```python
from build123d import *

# Parameters (mm, degrees)
BOSS_EXTRU_1_DEPTH   = 635
ESQUISSE2_R          = 486.41
BOSS_EXTRU_2_DEPTH   = 203.2
PER_AGE1_D           = 139.7
PER_AGE1_DEPTH       = 838.2
PER_AGE1_CBORE_D     = 266.7
PER_AGE1_CBORE_DEPTH = 165.1
PER_AGE2_D           = 139.7
PER_AGE2_DEPTH       = 838.2
PER_AGE2_CBORE_D     = 292.1
PER_AGE2_CBORE_DEPTH = 165.1


with BuildPart() as part:
    # Esquisse1 → Boss.-Extru.1 (new body)
    with BuildSketch(Plane.XY.offset(838.2)):
        with BuildLine():
            ThreePointArc((-720.101782381, 451.601786597), (-655.471932336, 350.063866609), (-659.625858178, 229.773752251))
            ThreePointArc((-659.625858178, 229.773752251), (-493.914086659, -493.914086659), (229.773752251, -659.625858178))
            ThreePointArc((229.773752251, -659.625858178), (350.063866609, -655.471932336), (451.601786597, -720.101782381))
            ThreePointArc((451.601786597, -720.101782381), (731.603841816, -731.603841816), (720.101782381, -451.601786597))
            ThreePointArc((720.101782381, -451.601786597), (655.471932336, -350.063866609), (659.625858178, -229.773752251))
            ThreePointArc((659.625858178, -229.773752251), (493.914086659, 493.914086659), (-229.773752251, 659.625858178))
            ThreePointArc((-229.773752251, 659.625858178), (-350.063866609, 655.471932336), (-451.601786597, 720.101782381))
            ThreePointArc((-451.601786597, 720.101782381), (-731.603841816, 731.603841816), (-720.101782381, 451.601786597))
        make_face()
    extrude(amount=-BOSS_EXTRU_1_DEPTH)

    # Esquisse2 → Boss.-Extru.2 (add)
    with BuildSketch(Plane(origin=(0, 0, 203.2), x_dir=(-1, 0, 0), z_dir=(0, 0, -1))):
        Circle(ESQUISSE2_R)
    extrude(amount=BOSS_EXTRU_2_DEPTH)

    # Perçage1
    with Locations(Plane.XY.offset(838.2)):
        with Locations((-596.9, 596.9)):
            CounterBoreHole(PER_AGE1_D / 2, PER_AGE1_CBORE_D / 2, PER_AGE1_CBORE_DEPTH, depth=PER_AGE1_DEPTH)

    # Perçage2
    with Locations(Plane.XY.offset(838.2)):
        with Locations((596.9, -596.9)):
            CounterBoreHole(PER_AGE2_D / 2, PER_AGE2_CBORE_D / 2, PER_AGE2_CBORE_DEPTH, depth=PER_AGE2_DEPTH)


solid = part.part
```
Input: part model. Units: mm. Frame: model coordinates. A direction names the side the tool comes from. Coordinates: 2 decimals unless noted, no trailing zeros. Write each loop counter-clockwise with the first axis right and the second up, starting at its lowest first coordinate (ties: lowest second). Pieces come first, ordered by that corner, then holes.
1) Section A-A on x = 0. Output: boundary loops of the cut face in (y, z).
2) Section B-B on y = 596.9. Output: boundary loops of the cut face in (x, z), and give its area (3 significant figures).
3) Mould query, pull axis Y, two halves, no side actions, for faces 1 (the cylindrical face through (-728.451, 734.685, 525.145)), 2 (the flat face through (7, 7, 0)), 3 (the cylindrical face through (666.682, -593.829, 434.861)). Classes: pulls with the +Y half, pulls with the -Y half, needs draft (parallel to the pull), parting line crosses it, or undercut.
4) Set-up query: faces 4 (the cylindrical face through (-348.41, 655.03, 525.14)), 5 (the flat face through (339, 361, 203.2)), 6 (the cylindrical face through (-469.708, 636.955, 756.806)). Return all of +Z, -Z, +X, -X, +Y, -Y with unobstructed straight access to the full face (end or side cutting, diameter ignored); none if empty.
5) Section C-C on z = 319. Output: boundary loops of the cut face in (x, y).
6) Material intervals for line 1 along Z through (x, y) = (-241, 445); line 2 along Z through (x, y) = (506, -585); line 3 along Y through (x, z) = (-596.9, 488.5), sorted ascending.
7) Pin query (flat end, axial travel): pin 1 Ø3 at (x, z) = (361, 549) entering from +Y; pin 2 Ø8 at (x, y) = (134, 495.5) entering from -Z; pin 3 Ø8 at (x, z) = (572, 394) entering from +Y. Return the tip coordinate at first contact, or that it passes through.
Check result:
1. outline: (-698.5, 203.2) - (-486.41, 203.2) - (-486.41, 0) - (486.41, 0) - (486.41, 203.2) - (698.5, 203.2) - (698.5, 838.2) - (-698.5, 838.2) - close
2. outline: (-787.4, 203.2) - (-666.75, 203.2) - (-666.75, 673.1) - (-730.25, 673.1) - (-730.25, 838.2) - (-787.4, 838.2) - close; (-527.05, 203.2) - (362.78, 203.2) - (362.78, 838.2) - (-463.55, 838.2) - (-463.55, 673.1) - (-527.05, 673.1) - close
2. area: 621,000 mm2
3. face 1: parting line crosses it
3. face 2: needs draft
3. face 3: undercut
4. face 4: +Z, -Z, +Y
4. face 5: -Z
4. face 6: +Z
5. outline: (-720.1, 451.6) arc R203.2 cw to (-659.63, 229.77) arc R698.5 ccw to (229.77, -659.63) arc R203.2 cw to (451.6, -720.1) arc R190.5 ccw (long way) to (720.1, -451.6) arc R203.2 cw to (659.63, -229.77) arc R698.5 ccw to (-229.77, 659.63) arc R203.2 cw to (-451.6, 720.1) arc R190.5 ccw (long way) to start; hole circle Ø139.7 at (-596.9, 596.9); hole circle Ø139.7 at (596.9, -596.9)
6. line 1: z = 203.2 to 838.2
6. line 2: z = 203.2 to 673.1
6. line 3: y = -362.78 to 527.05, 666.75 to 787.4
7. pin 1: stops at y = 598.88
7. pin 2: stops at z = 203.2
7. pin 3: stops at y = 406.54
